Here's how the part is built. I have some questions about the finished solid (model axes, mm). Face numbers are marked on the shaded views. A direction names the side the tool comes from. Round coordinates to 2 decimals unless told otherwise and drop trailing zeros. Write each loop counter-clockwise with the first axis right and the second up, starting at its lowest first coordinate (ties: lowest second). Pieces come first, ordered by that corner, then holes. Notation, with made-up numbers: (-34.5, -10) - (-26.5, -10) arc R19 ccw to (-26.5, 25) - close; hole circle Ø8 at (53.25, 16.25). An arc over 180 degrees is marked (long way). One line per question, with ' | ' between items. Start each with the question number.
(1) Thinking about a two-plate mould opening in Z: for the marked faces 1, 2 and 3, which applies, pulls with the +Z half, pulls with the -Z half, needs draft (parallel to the pull), parting line crosses it, or undercut?
(2) Imagine slicing it at C-C (x = 0). Write out the boundary of the cut face in (y, z).
(3) For the marked faces 4 and 5, which set-ups out of +Z, -Z, +X, -X, +Y, -Y let a thin tool reach every point of the face, with its end or its side?
(4) Imagine slicing it at A-A (y = 6.75). Write out the boundary of the cut face in (x, z).
(5) Imagine slicing it at D-D (x = 33.5). Write out the boundary of the cut face in (y, z), plus the area to 3 significant figures.
(6) Will these pins go through, and if not, where does the flat tip stop? pin 1 (10 mm diameter, centred on x = 40, z = -5.5, fed in from +Y); pin 2 (4 mm diameter, centred on y = 8, z = -37, fed in from +X); pin 3 (3 mm diameter, centred on x = -42.5, y = 13, fed in from +Z).
(7) Imagine slicing it at B-B (z = 0). Write out the boundary of the cut face in (x, y), plus the area to 3 significant figures.
(8) If I drill on L1, parallel to Z at x = 0, y = 13; L2, parallel to Y at x = -29, z = -32, over which ranges is the centre line in solid material (lowest first)?
from build123d import *

# Parameters (mm, degrees)
SKETCH1_R           = 60
BOSS_EXTRUDE1_DEPTH = 5
SKETCH2_R           = 50
BOSS_EXTRUDE2_DEPTH = 13.8
SKETCH3_R           = 47.5
CUT_EXTRUDE1_DEPTH  = 13.8
SKETCH4_R           = 7.5
BOSS_EXTRUDE3_DEPTH = 13.8
SKETCH6_R           = 3.25
CUT_EXTRUDE2_DEPTH  = 35


with BuildPart() as part:
    # Sketch1 → Boss-Extrude1 (new body)
    with BuildSketch(Plane(origin=(0, 0, 0), x_dir=(1, 0, 0), z_dir=(0, 1, 0))):
        Circle(SKETCH1_R)
    extrude(amount=BOSS_EXTRUDE1_DEPTH)

    # Sketch2 → Boss-Extrude2 (add)
    with BuildSketch(Plane(origin=(0, 5, 0), x_dir=(1, 0, 0), z_dir=(0, 1, 0))):
        Circle(SKETCH2_R)
    extrude(amount=BOSS_EXTRUDE2_DEPTH)

    # Sketch3 → Cut-Extrude1 (cut)
    with BuildSketch(Plane(origin=(0, 18.8, 0), x_dir=(1, 0, 0), z_dir=(0, 1, 0))):
        Circle(SKETCH3_R)
    extrude(amount=-CUT_EXTRUDE1_DEPTH, mode=Mode.SUBTRACT)

    # Sketch4 → Boss-Extrude3 (add)
    with BuildSketch(Plane(origin=(0, 5, 0), x_dir=(1, 0, 0), z_dir=(0, 1, 0))):
        Circle(SKETCH4_R)
    extrude(amount=BOSS_EXTRUDE3_DEPTH)

    # Sketch6 → Cut-Extrude2 (cut)
    with BuildSketch(Plane(origin=(0, 18.8, 0), x_dir=(1, 0, 0), z_dir=(0, 1, 0))):
        Circle(SKETCH6_R)
    extrude(amount=-CUT_EXTRUDE2_DEPTH, mode=Mode.SUBTRACT)


solid = part.part
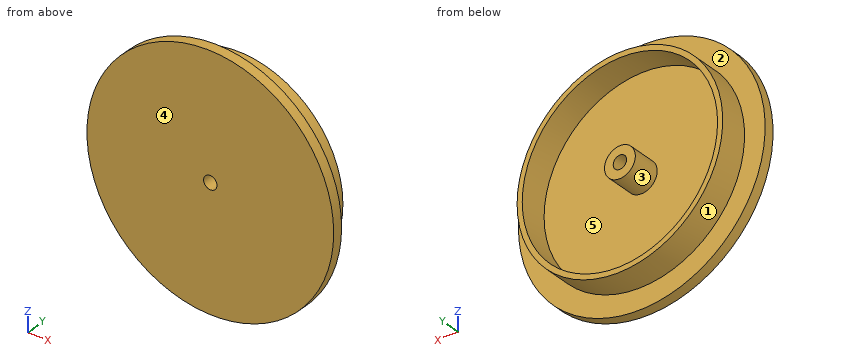
Check sheet entries:
1) face 1: parting line crosses it | face 2: needs draft | face 3: undercut
2) outline: (0, -60) - (5, -60) - (5, -50) - (18.8, -50) - (18.8, -47.5) - (5, -47.5) - (5, -7.5) - (18.8, -7.5) - (18.8, -3.25) - (0, -3.25) - close; (0, 3.25) - (18.8, 3.25) - (18.8, 7.5) - (5, 7.5) - (5, 47.5) - (18.8, 47.5) - (18.8, 50) - (5, 50) - (5, 60) - (0, 60) - close
3) face 4: +Z, -Z, +X, -X, -Y | face 5: +Y
4) outline: circle Ø100 at (0, 0); circle Ø15 at (0, 0); hole circle Ø95 at (0, 0); hole circle Ø6.5 at (0, 0)
5) outline: (0, -49.78) - (5, -49.78) - (5, -37.12) - (18.8, -37.12) - (18.8, -33.67) - (5, -33.67) - (5, 33.67) - (18.8, 33.67) - (18.8, 37.12) - (5, 37.12) - (5, 49.78) - (0, 49.78) - close | area: 593 mm^2
6) pin 1: y = 5 | pin 2: x = 35.71 | pin 3: z = 28.62
7) outline: (-60, 0) - (-3.25, 0) - (-3.25, 18.8) - (-7.5, 18.8) - (-7.5, 5) - (-47.5, 5) - (-47.5, 18.8) - (-50, 18.8) - (-50, 5) - (-60, 5) - close; (3.25, 0) - (60, 0) - (60, 5) - (50, 5) - (50, 18.8) - (47.5, 18.8) - (47.5, 5) - (7.5, 5) - (7.5, 18.8) - (3.25, 18.8) - close | area: 754 mm^2
8) L1: -50 to -47.5, -7.5 to -3.25, 3.25 to 7.5, 47.5 to 50 | L2: 0 to 5
